Read the model definition and answer for the solid it produces. Units are mm, in the model's axes. A direction names the side the tool comes from. Round coordinates to 2 decimals unless told otherwise and drop trailing zeros. Write each loop counter-clockwise with the first axis right and the second up, starting at its lowest first coordinate (ties: lowest second). Pieces come first, ordered by that corner, then holes. Notation, with made-up numbers: M 59.25,49.5 L 98.25,49.5 A28 ccw 98.25,78.5 Z; hole C 28,77.25 d10. An arc over 180 degrees is marked long. Use one line per item in the form item = value. Start each with the question number.
```python
from build123d import *

# Parameters (mm, degrees)
CORTAR_EXTRUIR1_DEPTH = 113.54200331


with BuildPart() as part:
    # Croquis2 → Revolución1 (revolve)
    with BuildSketch(Plane.XY, mode=Mode.PRIVATE) as revoluci_n1_sk:
        with BuildLine():
            Line((4.7625, 95.25), (12.7, 95.25))
            Line((12.7, 95.25), (12.7, 112.95))
            add(Edge.make_bspline(
                [(12.7, 112.95), (18.502741551, 112.95), (18.502741551, 107.95)],
                knots=[0, 0, 0, 1, 1, 1], degree=2))
            Line((18.502741551, 107.95), (22.5, 107.95))
            Line((22.5, 107.95), (22.5, 110.964889394))
            add(Edge.make_bspline(
                [(7.5, 127.95), (17.074954072, 127.95), (22.5, 119.467155594), (22.5, 110.964889394)],
                knots=[0, 0, 0, 0, 1, 1, 1, 1], degree=3))
            Line((7.5, 127.95), (7.5, 115.25))
            Line((7.5, 115.25), (0, 115.25))
            Line((0, 115.25), (0, 0))
            Line((0, 0), (4.7625, 0))
            Line((4.7625, 0), (4.7625, 95.25))
        make_face()
    revolve(revoluci_n1_sk.sketch.rotate(Axis((0, 0, 0), (0, 1, 0)), 90), axis=Axis((0, 0, 0), (0, 1, 0)))

    # Croquis3 → Cortar-Extruir1 (cut, through all)
    with BuildSketch(Plane.XZ.offset(-107.95)):
        with BuildLine():
            ThreePointArc((20.772727273, 8.645449766), (19.5, 0), (20.772727273, -8.645449766))
            ThreePointArc((20.772727273, -8.645449766), (22.5, 0), (20.772727273, 8.645449766))
        make_face()
        with BuildLine():
            ThreePointArc((17.873542761, -13.666984641), (9.75, -16.887495374), (2.899184512, -22.312434407))
            ThreePointArc((2.899184512, -22.312434407), (11.25, -19.485571585), (17.873542761, -13.666984641))
        make_face()
        with BuildLine():
            ThreePointArc((-2.899184512, -22.312434407), (-9.75, -16.887495374), (-17.873542761, -13.666984641))
            ThreePointArc((-17.873542761, -13.666984641), (-11.25, -19.485571585), (-2.899184512, -22.312434407))
        make_face()
        with BuildLine():
            ThreePointArc((-20.772727273, -8.645449766), (-19.5, 0), (-20.772727273, 8.645449766))
            ThreePointArc((-20.772727273, 8.645449766), (-22.5, 0), (-20.772727273, -8.645449766))
        make_face()
        with BuildLine():
            ThreePointArc((-17.873542761, 13.666984641), (-9.75, 16.887495374), (-2.899184512, 22.312434407))
            ThreePointArc((-2.899184512, 22.312434407), (-11.25, 19.485571585), (-17.873542761, 13.666984641))
        make_face()
        with BuildLine():
            ThreePointArc((2.899184512, 22.312434407), (9.75, 16.887495374), (17.873542761, 13.666984641))
            ThreePointArc((17.873542761, 13.666984641), (11.25, 19.485571585), (2.899184512, 22.312434407))
        make_face()
    extrude(amount=-CORTAR_EXTRUIR1_DEPTH, mode=Mode.SUBTRACT)


solid = part.part
```
Q1. Each of these flat-tipped pins is pushed along its axis until it touches: pin 1 Ø2 at (x, y) = (10, 112.5) entering from -Z; pin 2 Ø9 at (x, z) = (0, 0) entering from +Y; pin 3 Ø12 at (x, y) = (3.5, 65.5) entering from +Z. Where does it stop, or does it pass through?
Q2. Straight lines are drawn through the part: line 1 (X direction, y = 119.5, z = 0); line 2 (Y direction, x = 17, z = -9.5); line 3 (X direction, y = 121.5, z = 0). For each, find the intervals that lie inside material, in ascending order. Write a range as [from, to].
Q3. For a pull along X with two mould halves and no side action, classify faces 4 (the face through (-19.51, 109.48, 11.21)), 5 (the face through (-6.324, 121.511, -4.032)), 6 (the face through (4.65, 48.29, 1.03)) as +X half, -X half, draft (parallel to the pull), parting line (faces both ways), or undercut.
Q4. A tool of negligible diameter and unlimited length cuts with its end or side. For faces 1 (the face through (0, 115.25, 0)), 2 (the face through (-3.2, 107.95, -18.4)), 3 (the face through (0, 0, 0)), from which of +Z, -Z, +X, -X, +Y, -Y can it reach the whole face along a straight path? Write none if from no direction.
Q5. Find section A-A on y = 52. Write down the section's boundary in (x, z) (1 decimal).
Response:
q1.pin_1 = -17.34
q1.pin_2 = 115.25
q1.pin_3 = 4.76
q2.line_1 = [-19.5, -7.5], [7.5, 19.5]
q2.line_2 = [107.95, 121.43]
q2.line_3 = [-19.43, -7.5], [7.5, 19.43]
q3.face_4 = -X half
q3.face_5 = undercut
q3.face_6 = parting line
q4.face_1 = +Y
q4.face_2 = -Y
q4.face_3 = +Z, -Z, +X, -X, -Y
q5.outline = C 0,0 d9.5
